Part print with two shaded views. Sizes in mm from the minimum x, y, z corner. Coordinates: 2 decimals unless noted, no trailing zeros. Write each loop counter-clockwise with the first axis right and the second up, starting at its lowest first coordinate (ties: lowest second). Pieces come first, ordered by that corner, then holes. Notation, with made-up numbers: (19, 85) - (52, 85) arc R15 ccw to (52, 101) - close; hole circle Ø4 at (48, 14.5). An arc over 180 degrees is marked (long way). Answer in a Markdown table with one row per item. Add a question column.
Q1. Band-saw the part on B-B (y = 66). List the corners of the cut face in (x, z) (1 decimal), and give its area (3 significant figures).
Q2. Pin check, flat tip, straight feed: pin 1 (1.5 mm diameter, centred on x = 5, y = 48.5, fed in from -Z). Stop position of the tip, or through.
Q3. Band-saw the part on A-A (x = 7.5). List the corners of the cut face in (y, z) (1 decimal).
Q4. Two-plate mould, pull along Z, no slides. Class the marked faces 1, 2, 3 and 4: +Z half, -Z half, draft (parallel to the pull), parting line (faces both ways), or undercut.
Q5. Drill centre lines: line 1 along Y through (x, z) = (3, 12); line 2 along Y through (x, z) = (4, 12.5); line 3 along Z through (x, y) = (4.25, 39) (1 decimal). Where is each one in solid material? Low to high. Write a range as from..to.
Q6. Band-saw the part on C-C (z = 14). List the corners of the cut face in (x, y), and give its area (3 significant figures).
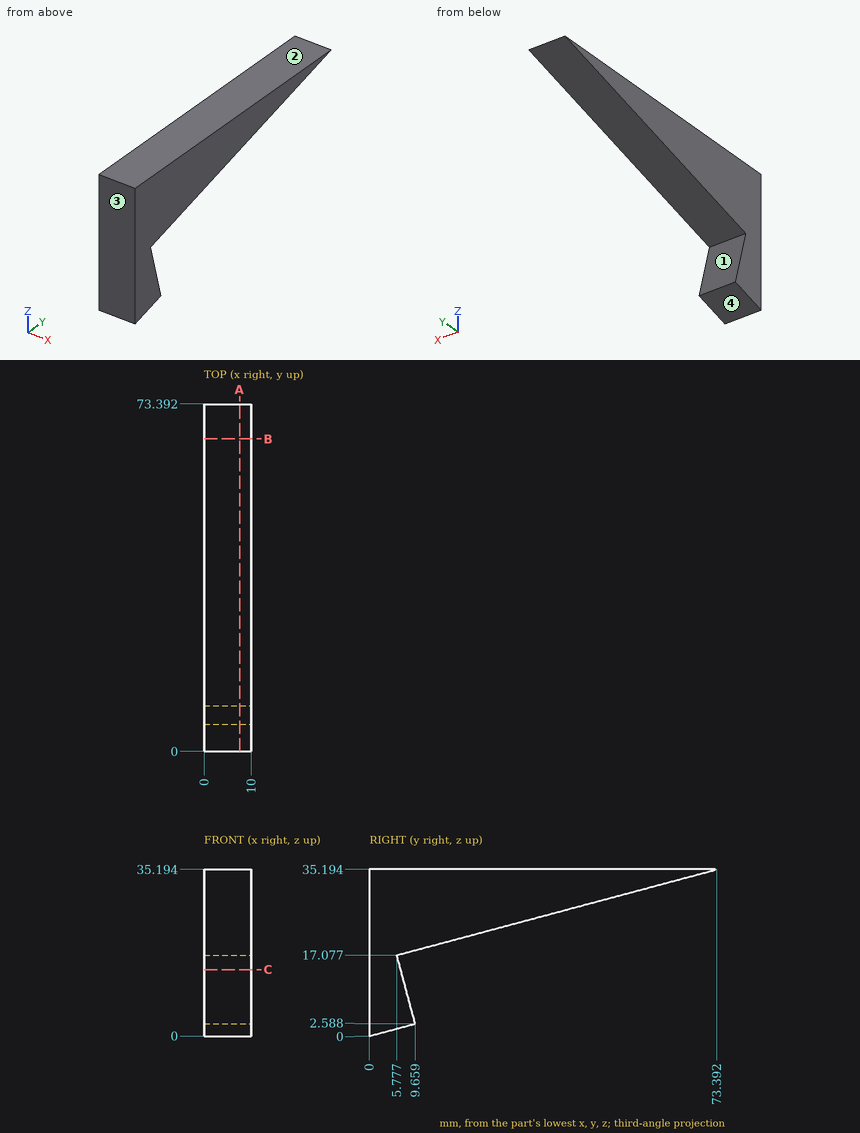
Checked values:
| question | item | result |
|---|---|---|
| 1 | outline | (0, 33.2) - (10, 33.2) - (10, 35.2) - (0, 35.2) - close |
| 1 | area | 19.8 mm² |
| 2 | pin 1 | stops at z = 28.32 |
| 3 | outline | (0, 0) - (9.7, 2.6) - (5.8, 17.1) - (73.4, 35.2) - (0, 35.2) - close |
| 4 | face 1 | undercut |
| 4 | face 2 | +Z half |
| 4 | face 3 | draft |
| 4 | face 4 | -Z half |
| 5 | line 1 | y = 0..7.14 |
| 5 | line 2 | y = 0..7 |
| 5 | line 3 | z = 26..35.2 |
| 6 | outline | (0, 0) - (10, 0) - (10, 6.6) - (0, 6.6) - close |
| 6 | area | 66.0 mm² |
